Geometry check sheet. Reference: the model listing, model coordinates, mm. Coordinates: 2 decimals unless noted, no trailing zeros. Write each loop counter-clockwise with the first axis right and the second up, starting at its lowest first coordinate (ties: lowest second). Pieces come first, ordered by that corner, then holes. Notation, with made-up numbers: (-38, 44.5) -> (-9, 44.5) arc R17 cw to (-9, 52.5) -> close; hole circle Ø4 at (-11.5, 45.25). An arc over 180 degrees is marked (long way). Answer in a Markdown table with one row per item. Add a question column.
1. Cross-section at C-C on x = -30. Record the cut outline in (y, z), and give its area (3 significant figures).
2. Scan lines: L1, parallel to Y at x = -30, z = 2.35; L2, parallel to X at y = -49.5, z = 1.55; L3, parallel to Y at x = 10, z = 2.85. Record each from-to range of solid material in increasing order. Write a range as from..to.
3. Cross-section at D-D on y = -45. Record the cut outline in (x, z), and give its area (3 significant figures).
4. Cross-section at A-A on y = -90. Record the cut outline in (x, z).
5. Cross-section at B-B on z = 2.05. Give the number of separate pieces and of enclosed holes in the cut face, and give its area (3 significant figures).
```python
from build123d import *

# Parameters (mm, degrees)
SKETCH1_W           = 120
SKETCH1_H           = 200
BOSS_EXTRUDE1_DEPTH = 3
FILLET1_R           = 60
CUT_EXTRUDE1_DEPTH  = 3
SKETCH3_R           = 2
CUT_EXTRUDE2_DEPTH  = 10


with BuildPart() as part:
    # Sketch1 → Boss-Extrude1 (new body)
    with BuildSketch(Plane.XY):
        Rectangle(SKETCH1_W, SKETCH1_H)
    extrude(amount=BOSS_EXTRUDE1_DEPTH)

    # Fillet1
    fillet1_edges = [part.edges().sort_by_distance(p)[0] for p in [
        (60, 100, 1.5),
        (-60, 100, 1.5),
    ]]
    fillet(fillet1_edges, radius=FILLET1_R - 0.0001)  # a hair under: the kernel refuses the full size

    # Sketch2 → Cut-Extrude1 (cut)
    with BuildSketch(Plane.XY.offset(3)):
        with BuildLine():
            Line((-35.5, -16), (35.5, -16))
            ThreePointArc((35.5, -16), (37.621320344, -16.878679656), (38.5, -19))
            Line((38.5, -19), (38.5, -51))
            ThreePointArc((38.5, -51), (37.621320344, -53.121320344), (35.5, -54))
            Line((35.5, -54), (-35.5, -54))
            ThreePointArc((-35.5, -54), (-37.621320344, -53.121320344), (-38.5, -51))
            Line((-38.5, -51), (-38.5, -19))
            ThreePointArc((-38.5, -19), (-37.621320344, -16.878679656), (-35.5, -16))
        make_face()
    extrude(amount=-CUT_EXTRUDE1_DEPTH, mode=Mode.SUBTRACT)

    # Sketch3 → Cut-Extrude2 (cut)
    with BuildSketch(Plane.XY.offset(3)):
        with Locations((-30, -90)):
            Circle(SKETCH3_R)
        with Locations((-30, 10)):
            Circle(SKETCH3_R)
        with Locations((30, 10)):
            Circle(SKETCH3_R)
        with Locations((30, -90)):
            Circle(SKETCH3_R)
    extrude(amount=-CUT_EXTRUDE2_DEPTH, mode=Mode.SUBTRACT)


solid = part.part
```
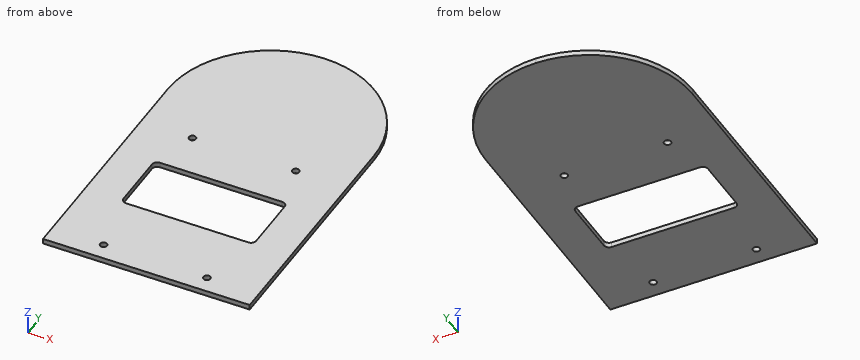
Results found:
| question | item | result |
|---|---|---|
| 1 | outline | (-100, 0) -> (-92, 0) -> (-92, 3) -> (-100, 3) -> close; (-88, 0) -> (-54, 0) -> (-54, 3) -> (-88, 3) -> close; (-16, 0) -> (8, 0) -> (8, 3) -> (-16, 3) -> close; (12, 0) -> (91.96, 0) -> (91.96, 3) -> (12, 3) -> close |
| 1 | area | 438 mm^2 |
| 2 | L1 | y = -100..-92, -88..-54, -16..8, 12..91.96 |
| 2 | L2 | x = -60..-38.5, 38.5..60 |
| 2 | L3 | y = -100..-54, -16..99.16 |
| 3 | outline | (-60, 0) -> (-38.5, 0) -> (-38.5, 3) -> (-60, 3) -> close; (38.5, 0) -> (60, 0) -> (60, 3) -> (38.5, 3) -> close |
| 3 | area | 129 mm^2 |
| 4 | outline | (-60, 0) -> (-32, 0) -> (-32, 3) -> (-60, 3) -> close; (-28, 0) -> (28, 0) -> (28, 3) -> (-28, 3) -> close; (32, 0) -> (60, 0) -> (60, 3) -> (32, 3) -> close |
| 5 | separate pieces | 1 |
| 5 | enclosed holes | 5 |
| 5 | area | 19,500 mm^2 |
